For this review, take the finished solid that the model builds, in its own axes (mm). Face numbers are marked on the shaded views. A direction names the side the tool comes from. Give positions to 0.01 mm unless a question says otherwise; leave off trailing zeros. One line per question, with ' | ' between items. Start each with the question number.
(1) Insertion check: P1, Ø4, axis at x = 69.33, z = 66.31, coming from the +Y side (3 decimals); P2, Ø4, axis at x = 82.28, z = 59.45, coming from the -Y side (3 decimals). Each pin has a flat end and moves straight along its axis. Give the tip position at first contact, or say it passes through.
(2) Consider section A-A (y = 5). Give the number of separate pieces and of enclosed holes in the cut face, and give its area (3 significant figures).
(3) Wall thickness on probe 1 along Z at (x, y) = (76.5, 5.75) (1 decimal); probe 2 along Z at (x, y) = (75, 3.5) (3 decimals); probe 3 along X at (y, z) = (4.75, 58.5): over which ranges is each line inside the solid? List them lowest first.
(4) Tool access review of the marked faces 1 and 2: name each direction out of +Z, -Z, +X, -X, +Y, -Y from which nothing blocks a thin tool from reaching the whole face with its end or side.
from build123d import *

# Parameters (mm, degrees)
BOSS_EXTRUDE1_DEPTH = 6.35
SKETCH3_R           = 1.5
CUT_EXTRUDE1_DEPTH  = 6.35
LPATTERN2_COUNT     = 22
LPATTERN2_PITCH     = 6.096
SKETCH4_R           = 1.5
CUT_EXTRUDE2_DEPTH  = 6.35
LPATTERN3_COUNT     = 16
LPATTERN3_PITCH     = 6.096
SKETCH6_W           = 120.396
SKETCH6_H           = 3.175
CUT_EXTRUDE3_DEPTH  = 12.192
SKETCH10_W          = 12.192
SKETCH10_H          = 12.192
CUT_EXTRUDE9_DEPTH  = 12.192
SKETCH9_W           = 146.304
SKETCH9_H           = 3.175
CUT_EXTRUDE8_DEPTH  = 12.192
SKETCH11_R          = 1.5
CUT_EXTRUDE10_DEPTH = 6.35
SKETCH13_R          = 1.5
CUT_EXTRUDE12_DEPTH = 6.35


with BuildPart() as part:
    # Sketch2 → Boss-Extrude1 (new body)
    with BuildSketch(Plane(origin=(0, 0, 0), x_dir=(1, 0, 0), z_dir=(0, 1, 0))):
        Polygon((-55.206688966, 44.945004491), (-73.167201208, 26.984492248), (-73.167201208, -75.450995509), (85.328798792, -75.450995509), (85.328798792, 44.945004491), align=None)
    extrude(amount=BOSS_EXTRUDE1_DEPTH)

    # Sketch3 → Cut-Extrude1 (cut)
    with BuildSketch(Plane(origin=(0, 6.35, 0), x_dir=(1, 0, 0), z_dir=(0, 1, 0))):
        with Locations(Location((82.280798792, 41.135004491, 0), (0, 0, 270))):
            Circle(SKETCH3_R)
    cut_extrude1 = extrude(amount=-CUT_EXTRUDE1_DEPTH, mode=Mode.SUBTRACT)

    # LPattern2: Cut-Extrude1 ×22
    with Locations(*[(-i * LPATTERN2_PITCH, 0, 0) for i in range(1, LPATTERN2_COUNT)]):
        add(cut_extrude1, mode=Mode.SUBTRACT)

    # Sketch4 → Cut-Extrude2 (cut)
    with BuildSketch(Plane(origin=(0, 6.35, 0), x_dir=(1, 0, 0), z_dir=(0, 1, 0))):
        with Locations(Location((-69.357201208, -72.402995509, 0), (0, 0, 270))):
            Circle(SKETCH4_R)
    cut_extrude2 = extrude(amount=-CUT_EXTRUDE2_DEPTH, mode=Mode.SUBTRACT)

    # LPattern3: Cut-Extrude2 ×16
    with Locations(*[(0, 0, -i * LPATTERN3_PITCH) for i in range(1, LPATTERN3_COUNT)]):
        add(cut_extrude2, mode=Mode.SUBTRACT)

    # Sketch6 → Cut-Extrude3 (cut)
    with BuildSketch(Plane(origin=(85.328798792, 0, 0), x_dir=(0, 0, -1), z_dir=(1, 0, 0))):
        with Locations((-15.252995509, 1.5875)):
            Rectangle(SKETCH6_W, SKETCH6_H)
    extrude(amount=-CUT_EXTRUDE3_DEPTH, mode=Mode.SUBTRACT)

    # Sketch10 → Cut-Extrude9 (cut)
    with BuildSketch(Plane(origin=(0, 6.35, 0), x_dir=(1, 0, 0), z_dir=(0, 1, 0))):
        with Locations((79.232798792, -69.354995509)):
            Rectangle(SKETCH10_W, SKETCH10_H)
    extrude(amount=-CUT_EXTRUDE9_DEPTH, mode=Mode.SUBTRACT)

    # Sketch9 → Cut-Extrude8 (cut)
    with BuildSketch(Plane.XY.offset(75.450995509)):
        with Locations((-0.015201208, 4.7625)):
            Rectangle(SKETCH9_W, SKETCH9_H)
    extrude(amount=-CUT_EXTRUDE8_DEPTH, mode=Mode.SUBTRACT)

    # Sketch11 → Cut-Extrude10 (cut)
    with BuildSketch(Plane(origin=(0, 6.35, 0), x_dir=(1, 0, 0), z_dir=(0, 1, 0))):
        with Locations(Location((82.280798792, -59.448995509, 0), (0, 0, 270))):
            Circle(SKETCH11_R)
        with Locations(Location((76.184798792, -59.448995509, 0), (0, 0, 270))):
            Circle(SKETCH11_R)
        with Locations(Location((69.326798792, -66.306995509, 0), (0, 0, 270))):
            Circle(SKETCH11_R)
        with Locations(Location((69.326798792, -72.402995509, 0), (0, 0, 270))):
            Circle(SKETCH11_R)
    extrude(amount=-CUT_EXTRUDE10_DEPTH, mode=Mode.SUBTRACT)

    # Sketch13 → Cut-Extrude12 (cut)
    with BuildSketch(Plane(origin=(0, 6.35, 0), x_dir=(1, 0, 0), z_dir=(0, 1, 0))):
        with Locations(Location((-59.337606782, 35.425933002, 0), (0, 0, 270))):
            Circle(SKETCH13_R)
        with Locations(Location((-55.027083843, 39.73645594, 0), (0, 0, 270))):
            Circle(SKETCH13_R)
        with Locations(Location((-63.64812972, 31.115410064, 0), (0, 0, 270))):
            Circle(SKETCH13_R)
        with Locations(Location((-67.958652658, 26.804887126, 0), (0, 0, 270))):
            Circle(SKETCH13_R)
    extrude(amount=-CUT_EXTRUDE12_DEPTH, mode=Mode.SUBTRACT)


solid = part.part
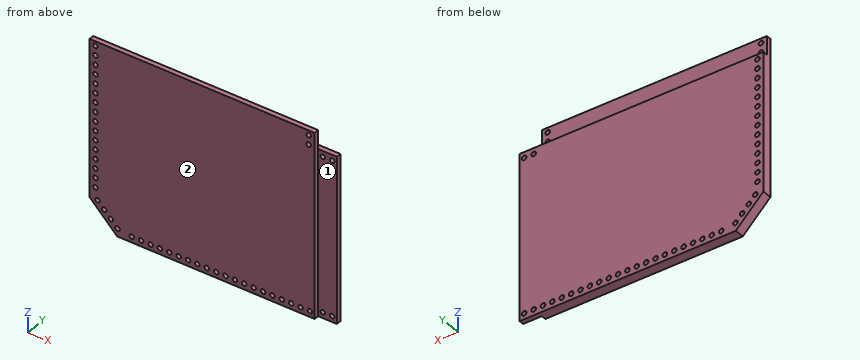
A:
1) P1: stops at y = 3.175 | P2: stops at y = 3.175
2) separate pieces: 1 | enclosed holes: 42 | area: 16,700 mm^2
3) probe 1: z = -44.9 to -42.6, -39.7 to 58, 60.9 to 63.3 | probe 2: z = -44.945 to -42.055, -40.215 to 58.529, 60.369 to 63.259 | probe 3: x = -73.17 to 75.02, 77.35 to 81.12, 83.44 to 85.33
4) face 1: +Z, -Z, +X, -Y | face 2: +Z, -Z, +X, -X, -Y
